from build123d import *

# Parameters (mm, degrees)
BOSS_EXTRUDE1_DEPTH = 44
CUT_EXTRUDE1_DEPTH  = 45
SKETCH2_W           = 24
SKETCH2_H           = 44
SKETCH2_W_2         = 21
SKETCH2_H_2         = 41
BOSS_EXTRUDE2_DEPTH = 15
SKETCH2_2_W         = 21
SKETCH2_2_H         = 41
BOSS_EXTRUDE3_DEPTH = 3


with BuildPart() as part:
    # Sketch1 → Boss-Extrude1 (new body)
    with BuildSketch(Plane.XY):
        with BuildLine():
            Line((-12, 0), (12, 0))
            Line((12, 0), (18.464466094, -6.464466094))
            ThreePointArc((18.464466094, -6.464466094), (19.548329851, -11.913417162), (14.928932188, -15))
            Line((14.928932188, -15), (-14.928932188, -15))
            ThreePointArc((-14.928932188, -15), (-19.548329851, -11.913417162), (-18.464466094, -6.464466094))
            Line((-18.464466094, -6.464466094), (-12, 0))
        make_face()
    extrude(amount=BOSS_EXTRUDE1_DEPTH)

    # Sketch3 → Cut-Extrude1 (cut, through all)
    with BuildSketch(Plane.XY.offset(44)):
        with BuildLine():
            Line((-14.928932188, -13.4), (14.928932188, -13.4))
            ThreePointArc((14.928932188, -13.4), (18.070122599, -11.30112367), (17.333095244, -7.595836944))
            Line((17.333095244, -7.595836944), (11.3372583, -1.6))
            Line((11.3372583, -1.6), (-11.3372583, -1.6))
            Line((-11.3372583, -1.6), (-17.333095244, -7.595836944))
            ThreePointArc((-17.333095244, -7.595836944), (-18.070122599, -11.30112367), (-14.928932188, -13.4))
        make_face()
    extrude(amount=-CUT_EXTRUDE1_DEPTH, mode=Mode.SUBTRACT)

    # Sketch2 → Boss-Extrude2 (add)
    with BuildSketch(Plane(origin=(0, 0, 0), x_dir=(1, 0, 0), z_dir=(0, 1, 0))):
        with Locations((0, -22)):
            Rectangle(SKETCH2_W, SKETCH2_H)
        with Locations((0, -22)):
            Rectangle(SKETCH2_W_2, SKETCH2_H_2, mode=Mode.SUBTRACT)
    extrude(amount=BOSS_EXTRUDE2_DEPTH)

    # Sketch2<2> → Boss-Extrude3 (add)
    with BuildSketch(Plane(origin=(0, 0, 0), x_dir=(1, 0, 0), z_dir=(0, 1, 0))):
        with Locations((0, -22)):
            Rectangle(SKETCH2_2_W, SKETCH2_2_H)
    extrude(amount=BOSS_EXTRUDE3_DEPTH)


solid = part.part
Work out the finished part from the listing and answer in its coordinate system (mm). A direction names the side the tool comes from. Coordinates: 2 decimals unless noted, no trailing zeros. Write each loop counter-clockwise with the first axis right and the second up, starting at its lowest first coordinate (ties: lowest second). Pieces come first, ordered by that corner, then holes.
1. Consider line 1 along Z through (x, y) = (7.5, 3.75); line 2 along Y through (x, z) = (7, 3); line 3 along X through (y, z) = (9.5, 15.5). Determine where each line is inside the solid, lowest interval first.
Results list:
line 1: z = 0 to 1.5, 42.5 to 44
line 2: y = -15 to -13.4, -1.6 to 3
line 3: x = -12 to -10.5, 10.5 to 12
2. The part is cut by section C-C, the plane y = -12.25. Write down the section's boundary in (x, z), and give its area (3 significant figures).
Results list:
outline: (-19.39, 0) - (-17.48, 0) - (-17.48, 44) - (-19.39, 44) - close; (17.48, 0) - (19.39, 0) - (19.39, 44) - (17.48, 44) - close
area: 169 mm2
3. The part is cut by section A-A, the plane z = 29. Write down the section's boundary in (x, y), and give its area (3 significant figures).
Results list:
outline: (-18.46, -6.46) arc R5 ccw to (-14.93, -15) - (14.93, -15) arc R5 ccw to (18.46, -6.46) - (12, 0) - (12, 15) - (10.5, 15) - (10.5, 3) - (-10.5, 3) - (-10.5, 15) - (-12, 15) - (-12, 0) - close; hole (-17.33, -7.6) arc R3.4 ccw to (-14.93, -13.4) - (14.93, -13.4) arc R3.4 ccw to (17.33, -7.6) - (11.34, -1.6) - (-11.34, -1.6) - close
area: 253 mm2
4. The part is cut by section B-B, the plane x = 9.5. Write down the section's boundary in (y, z).
Results list:
outline: (-15, 0) - (-13.4, 0) - (-13.4, 44) - (-15, 44) - close; (-1.6, 0) - (15, 0) - (15, 1.5) - (3, 1.5) - (3, 42.5) - (15, 42.5) - (15, 44) - (-1.6, 44) - close
5. The part is cut by section D-D, the plane y = 12. Write down the section's boundary in (x, z), and give its area (3 significant figures).
Results list:
outline: (-12, 0) - (12, 0) - (12, 44) - (-12, 44) - close; hole (-10.5, 1.5) - (10.5, 1.5) - (10.5, 42.5) - (-10.5, 42.5) - close
area: 195 mm2
6. Flat-ended cylindrical pins translate along their axes: pin 1 (6 mm diameter, centred on y = 8, z = 31.5, fed in from +X); pin 2 (9 mm diameter, centred on x = -1.5, z = 20.5, fed in from +Y); pin 3 (9.5 mm diameter, centred on y = 12, z = 27, fed in from -X). Find the tip coordinate at first contact, or state that the pin passes through.
Results list:
pin 1: stops at x = 12
pin 2: stops at y = 3
pin 3: stops at x = -12
7. For a pull along Y with two mould halves and no side action, classify faces 6 (the cylindrical face through (-18.09, -11.25, 22.31)), 7 (the flat face through (-10.5, 9, 22)), 8 (the flat face through (15, -3, 22)), 9 (the flat face through (-14.293, -4.556, 22.308)) as +Y half, -Y half, draft (parallel to the pull), parting line (faces both ways), or undercut.
Results list:
face 6: undercut
face 7: draft
face 8: +Y half
face 9: undercut
8. For faces 1 (the flat face through (-11, 15, 20)), 2 (the flat face through (12, 7, 22)), 3 (the flat face through (0, 3, 22)), 4 (the flat face through (0, -1.6, 22)), 5 (the flat face through (-12, 7, 22)), determine the directions among +Z, -Z, +X, -X, +Y, -Y from which every point of the face is accessible in a straight line to the end or side of a thin tool.
Results list:
face 1: +Z, -Z, +X, -X, +Y
face 2: +Z, -Z, +X, +Y
face 3: +Y
face 4: +Z, -Z
face 5: +Z, -Z, -X, +Y
